Could you check a few things on this model? Use its own coordinates, in mm. A direction names the side the tool comes from. Round coordinates to 2 decimals unless told otherwise and drop trailing zeros. Loops run counter-clockwise (first coordinate to the right, second up) from the corner with the lowest first, then second, coordinate; pieces in that order, holes last. Notation, with made-up numbers: (-22, -24) -> (20, -24) arc R12 cw to (20, -1) -> close; hole circle Ø7 at (-27, -8). An arc over 180 degrees is marked (long way). One line per item, written item: value.
```python
from build123d import *

# Parameters (mm, degrees)
F0_W           = 97
F0_H           = 150
F0_R           = 7.367785
F1_DEPTH       = 1.5
F3_D           = 2
F3_CSINK_D     = 4
F3_CSINK_ANGLE = 90
F5_D           = 2


# Not quite as in the source:
# - a feature names something its author has since deleted; it is built from what else it names


with BuildPart() as f1:
    # F0 (on Front) → F1 (new body)
    with BuildSketch(Plane.XZ):
        Rectangle(F0_W, F0_H)
        with BuildLine():
            Line((-31.5249225795, -7.60684), (-10.5249225795, -7.60684))
            ThreePointArc((-10.5249225795, -7.60684), (-5.5751751112, -9.6570925317), (-3.5249225795, -14.60684))
            Line((-3.5249225795, -14.60684), (-3.5249225795, -46))
            ThreePointArc((-3.5249225795, -46), (-5.5751751112, -50.9497474683), (-10.5249225795, -53))
            Line((-10.5249225795, -53), (-31.5249225795, -53))
            ThreePointArc((-31.5249225795, -53), (-36.4746700478, -50.9497474683), (-38.5249225795, -46))
            Line((-38.5249225795, -46), (-38.5249225795, -14.60684))
            ThreePointArc((-38.5249225795, -14.60684), (-36.4746700478, -9.6570925317), (-31.5249225795, -7.60684))
        make_face(mode=Mode.SUBTRACT)
        with BuildLine():
            ThreePointArc((38.5249225795, -46), (36.4746700478, -50.9497474683), (31.5249225795, -53))
            Line((31.5249225795, -53), (10.5249225795, -53))
            ThreePointArc((10.5249225795, -53), (5.5751751112, -50.9497474683), (3.5249225795, -46))
            Line((3.5249225795, -46), (3.5249225795, -14.60684))
            ThreePointArc((3.5249225795, -14.60684), (5.5751751112, -9.6570925317), (10.5249225795, -7.60684))
            Line((10.5249225795, -7.60684), (31.5249225795, -7.60684))
            ThreePointArc((31.5249225795, -7.60684), (36.4746700478, -9.6570925317), (38.5249225795, -14.60684))
            Line((38.5249225795, -14.60684), (38.5249225795, -46))
        make_face(mode=Mode.SUBTRACT)
        with BuildLine():
            ThreePointArc((-3.5249225795, 14.60684), (-5.5751751112, 9.6570925317), (-10.5249225795, 7.60684))
            Line((-10.5249225795, 7.60684), (-31.5249225795, 7.60684))
            ThreePointArc((-31.5249225795, 7.60684), (-36.4746700478, 9.6570925317), (-38.5249225795, 14.60684))
            Line((-38.5249225795, 14.60684), (-38.5249225795, 46))
            ThreePointArc((-38.5249225795, 46), (-36.4746700478, 50.9497474683), (-31.5249225795, 53))
            Line((-31.5249225795, 53), (-10.5249225795, 53))
            ThreePointArc((-10.5249225795, 53), (-5.5751751112, 50.9497474683), (-3.5249225795, 46))
            Line((-3.5249225795, 46), (-3.5249225795, 14.60684))
        make_face(mode=Mode.SUBTRACT)
        Circle(F0_R, mode=Mode.SUBTRACT)
        with BuildLine():
            ThreePointArc((10.5249225795, 7.60684), (5.5751751112, 9.6570925317), (3.5249225795, 14.60684))
            Line((3.5249225795, 14.60684), (3.5249225795, 46))
            ThreePointArc((3.5249225795, 46), (5.5751751112, 50.9497474683), (10.5249225795, 53))
            Line((10.5249225795, 53), (31.5249225795, 53))
            ThreePointArc((31.5249225795, 53), (36.4746700478, 50.9497474683), (38.5249225795, 46))
            Line((38.5249225795, 46), (38.5249225795, 14.60684))
            ThreePointArc((38.5249225795, 14.60684), (36.4746700478, 9.6570925317), (31.5249225795, 7.60684))
            Line((31.5249225795, 7.60684), (10.5249225795, 7.60684))
        make_face(mode=Mode.SUBTRACT)
    extrude(amount=F1_DEPTH)

    # F3 (through all)
    with Locations(Plane.XZ.offset(1.5)):
        with Locations((-43.5, -72), (43.5, -72), (43.5, 72), (-43.5, 72)):
            CounterSinkHole(F3_D / 2, F3_CSINK_D / 2, counter_sink_angle=F3_CSINK_ANGLE)

    # F5 (through all)
    with Locations(Plane.XZ.offset(1.5)):
        with Locations((-37, -73.5), (0, -73.5), (37, -73.5), (0, -11.5), (0, 50.5)):
            Hole(F5_D / 2)


solid = f1.part
```
Item 1: If we section it at B-B on z = 0: List the corners of the cut face in (x, y) for me, plus the area to 3 significant figures.
Output:
outline: (-48.5, -1.5) -> (-7.37, -1.5) -> (-7.37, 0) -> (-48.5, 0) -> close; (7.37, -1.5) -> (48.5, -1.5) -> (48.5, 0) -> (7.37, 0) -> close
area: 123 mm²
Item 2: I need wall thicknesses on line 1 (Z direction, x = 0, y = -0.3); line 2 (Z direction, x = -11, y = -0.55); line 3 (Z direction, x = 43.5, y = -0.25). Which ranges of each line are inside material? Lowest first, please. Write a range as from..to.
Output:
line 1: z = -75..-74.5, -72.5..-12.5, -10.5..-7.37, 7.37..49.5, 51.5..75
line 2: z = -75..-53, -7.61..7.61, 53..75
line 3: z = -75..-73, -71..71, 73..75
Item 3: If we section it at A-A on z = 31: List the corners of the cut face in (x, y) for me, plus the area to 3 significant figures.
Output:
outline: (-48.5, -1.5) -> (-38.52, -1.5) -> (-38.52, 0) -> (-48.5, 0) -> close; (-3.52, -1.5) -> (3.52, -1.5) -> (3.52, 0) -> (-3.52, 0) -> close; (38.52, -1.5) -> (48.5, -1.5) -> (48.5, 0) -> (38.52, 0) -> close
area: 40.5 mm²
Item 4: For faces 1 (the face through (-36.42, -0.74, 9.603)), 2 (the face through (42, -1, 72)), which set-ups out of +Z, -Z, +X, -X, +Y, -Y let a thin tool reach every point of the face, with its end or its side?
Output:
face 1: +Y, -Y
face 2: -Y
Item 5: Will this pin go through, and if not, where does the flat tip stop? pin 1 Ø2.5 at (x, z) = (43.5, 72) entering from +Y.
Output:
pin 1: stops at y = 0
